from build123d import *

# Parameters (mm, degrees)
BOSS_EXTRUDE1_DEPTH = 5
CUT_EXTRUDE1_START  = 11
SKETCH2_R           = 0.8
CUT_EXTRUDE1_DEPTH  = 23


with BuildPart() as part:
    # Sketch1 → Boss-Extrude1 (new body)
    with BuildSketch(Plane.XY):
        with BuildLine():
            Line((0, -11), (0, -3))
            Line((0, -3), (7, -3))
            Line((7, -3), (7, -4))
            Line((7, -4), (10, -4))
            Line((10, -4), (10, 6))
            Line((10, 6), (7, 6))
            Line((7, 6), (7, 5))
            Line((7, 5), (0, 5))
            Line((0, 5), (0, 12))
            ThreePointArc((0, 12), (-11.5, 0.5), (0, -11))
        make_face()
    extrude(amount=BOSS_EXTRUDE1_DEPTH)

    # Sketch2 → Cut-Extrude1 (cut, through all)
    with BuildSketch(Plane(origin=(0, 0, 0), x_dir=(1, 0, 0), z_dir=(0, 1, 0)).offset(CUT_EXTRUDE1_START)):
        with Locations((8.5, -2.5)):
            Circle(SKETCH2_R)
        with Locations((5.5, -2.5)):
            Circle(SKETCH2_R)
    extrude(amount=-CUT_EXTRUDE1_DEPTH, mode=Mode.SUBTRACT)


solid = part.part
For this review, take the finished solid that the model builds, in its own axes (mm). A direction names the side the tool comes from. Give positions to 0.01 mm unless a question says otherwise; leave off trailing zeros. Order: outer loops, then holes, each group sorted by start corner. A loop starts at its lowest first (then second) coordinate and runs counter-clockwise, first axis right, second up. Notation, with made-up numbers: (-35.75, 81) -> (6.25, 81) arc R28 cw to (6.25, 112) -> close; hole circle Ø7 at (19, 7.5). An arc over 180 degrees is marked (long way). Write item = value, one per line.
1) We need section B-B, the plane z = 2.5. Give the boundary of the cut face in (x, y), and give its area (3 significant figures).
Findings:
outline = (0, -11) -> (0, -3) -> (4.7, -3) -> (4.7, 5) -> (0, 5) -> (0, 12) arc R11.5 ccw to start; (6.3, -3) -> (7, -3) -> (7, -4) -> (7.7, -4) -> (7.7, 6) -> (7, 6) -> (7, 5) -> (6.3, 5) -> close; (9.3, -4) -> (10, -4) -> (10, 6) -> (9.3, 6) -> close
area = 265 mm^2
2) To check wall thickness, follow L1, parallel to X at y = 0.5, z = 2.5; L2, parallel to Z at x = 8.5, y = 0.25; L3, parallel to X at y = 1.5, z = 2.1. State the ranges of each line that lie inside material, in increasing order. Write a range as from..to.
Findings:
L1 = -11.5..4.7, 6.3..7.7, 9.3..10
L2 = 0..1.7, 3.3..5
L3 = -11.46..4.81, 6.19..7.81, 9.19..10
3) For faces 1 (the face through (7, -3.5, 2.5)), 2 (the face through (7.5, -4, 2.5)), 3 (the face through (4, 5, 2)), 4 (the face through (9.5, 6, 2.5)), list the 3-axis set-ups (+Z, -Z, +X, -X, +Y, -Y) from which the entire face can be reached by the end or side of a thin tool; tool diameter is ignored.
Findings:
face_1 = +Z, -Z, -Y
face_2 = +Z, -Z, +X, -Y
face_3 = +Z, -Z, +Y
face_4 = +Z, -Z, +X, +Y
4) We need section D-D, the plane y = 0.5. Give the boundary of the cut face in (x, z).
Findings:
outline = (-11.5, 0) -> (10, 0) -> (10, 5) -> (-11.5, 5) -> close; hole circle Ø1.6 at (5.5, 2.5); hole circle Ø1.6 at (8.5, 2.5)
5) We need section C-C, the plane z = 4.05. Give the boundary of the cut face in (x, y).
Findings:
outline = (0, -11) -> (0, -3) -> (7, -3) -> (7, -4) -> (10, -4) -> (10, 6) -> (7, 6) -> (7, 5) -> (0, 5) -> (0, 12) arc R11.5 ccw to start
6) Insertion check: pin 1 (2.5 mm diameter, centred on x = 8, z = 3.5, fed in from -Y); pin 2 (0.9 mm diameter, centred on x = 8.5, z = 2, fed in from +Y); pin 3 (2.5 mm diameter, centred on x = 5, z = 2, fed in from +Y); pin 4 (2 mm diameter, centred on x = 6, y = 7, fed in from +Z). Each pin has a flat end and moves straight along its axis. Give the tip position at first contact, or say it passes through.
Findings:
pin_1 = -4
pin_2 = 6
pin_3 = 5
pin_4 = through
7) We need section A-A, the plane x = 8.5. Give the boundary of the cut face in (y, z), and give its area (3 significant figures).
Findings:
outline = (-4, 0) -> (6, 0) -> (6, 1.7) -> (-4, 1.7) -> close; (-4, 3.3) -> (6, 3.3) -> (6, 5) -> (-4, 5) -> close
area = 34.0 mm^2
8) Draft analysis for pull direction Z (two halves, no side actions). For faces 5 (the face through (7.7, 1.1, 2.5)), 6 (the face through (10, 1, 2)), 7 (the face through (-1, 1, 0)), state which applies: pulls with the +Z half, pulls with the -Z half, needs draft (parallel to the pull), parting line crosses it, or undercut.
Findings:
face_5 = undercut
face_6 = needs draft
face_7 = pulls with the -Z half
